Source: CAD feature listing. Evaluate the final solid. Frame: model axes, mm. Face numbers are marked on the shaded views. Coordinates: 2 decimals unless noted, no trailing zeros. Order: outer loops, then holes, each group sorted by start corner. A loop starts at its lowest first (then second) coordinate and runs counter-clockwise, first axis right, second up. Notation, with made-up numbers: (-5, 19.5) -> (32, 19.5) arc R22 cw to (32, 46.5) -> close; hole circle Ø3 at (54.25, -21.5). An arc over 180 degrees is marked (long way). Put each result on its own line as item: value.
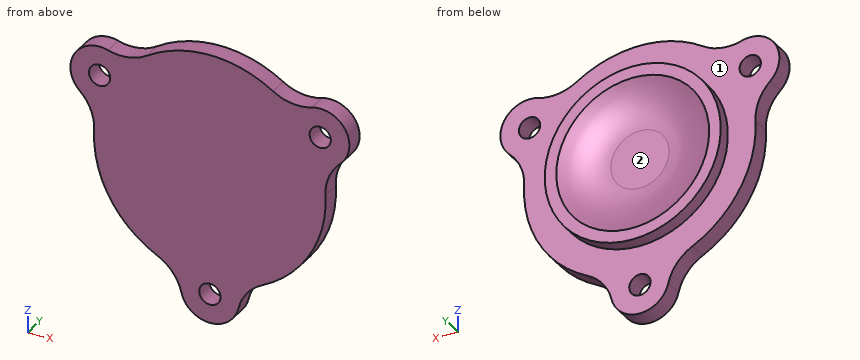
from build123d import *

# Parameters (mm, degrees)
SKETCH_1_R      = 12.5
EXTRUDE_1_DEPTH = 2
SKETCH_2_R      = 9.5
SKETCH_2_R_2    = 8.25
EXTRUDE_2_DEPTH = 1.4
FILLET_1_R      = 10
EXTRUDE_START   = -2
SKETCH_3_R      = 1.15
EXTRUDE_3_DEPTH = 2


with BuildPart() as part:
    # Эскиз1 → Бобышка-Вытянуть1 (new body)
    with BuildSketch(Plane(origin=(0, 0, 0), x_dir=(1, 0, 0), z_dir=(0, 1, 0))):
        with Locations(Location((0, 0, 0), (0, 0, 270))):
            Circle(SKETCH_1_R)
    extrude(amount=EXTRUDE_1_DEPTH)

    # Эскиз2 → Бобышка-Вытянуть2 (add)
    with BuildSketch(Plane(origin=(0, 2, 0), x_dir=(1, 0, 0), z_dir=(0, 1, 0))):
        with Locations(Location((0, 0, 0), (0, 0, 270))):
            Circle(SKETCH_2_R)
        with Locations(Location((0, 0, 0), (0, 0, 270))):
            Circle(SKETCH_2_R_2, mode=Mode.SUBTRACT)
    extrude(amount=EXTRUDE_2_DEPTH)

    # Скругление1
    # the kernel refuses this fillet: 10 mm, written as the material it adds along each edge
    with BuildSketch(Plane(origin=(0, 2, 0), x_dir=(0, 0, 1), z_dir=(-1, 0, 0))) as fillet_1_piece_1:
        with BuildLine():
            CenterArc((3.147059671, 10), FILLET_1_R, 270, 30.683417109)
            Line((3.147059671, 0), (3.147059671, -0.2))
            Line((3.147059671, -0.2), (8.25, -0.2))
            Line((8.25, -0.2), (8.45, 0))
            ThreePointArc((8.45, 0), (8.45, 0.7), (8.352058807, 1.228))
            Line((8.352058807, 1.228), (8.25, 1.4))
        make_face()
    revolve(axis=Axis((0, 2, 0), (0, 1, 0)))

    # Эскиз3 → Бобышка-Вытянуть3 (add)
    # profile 1 of 3: a face of its own
    with BuildSketch(Plane(origin=(0, 2, 0), x_dir=(1, 0, 0), z_dir=(0, 1, 0)).offset(EXTRUDE_START)):
        with BuildLine():
            ThreePointArc((5.670132274, 11.14), (0, 12.5), (-5.670132274, 11.14))
            ThreePointArc((-5.670132274, 11.14), (-4.001241708, 12.51371577), (-3.068132924, 14.463484663))
            ThreePointArc((-3.068132924, 14.463484663), (0, 16.9), (3.068132924, 14.463484663))
            ThreePointArc((3.068132924, 14.463484663), (4.001241708, 12.51371577), (5.670132274, 11.14))
        make_face()
        with Locations(Location((0, 13.75, 0), (0, 0, 270))):
            Circle(SKETCH_3_R, mode=Mode.SUBTRACT)
    # profile 2 of 3: a face of its own
    with BuildSketch(Plane(origin=(0, 2, 0), x_dir=(1, 0, 0), z_dir=(0, 1, 0)).offset(EXTRUDE_START)):
        with BuildLine():
            ThreePointArc((10.991678683, -9.888823385), (14.635829324, -8.45), (14.059811607, -4.574661277))
            ThreePointArc((14.059811607, -4.574661277), (12.837816607, -2.791680919), (12.482589135, -0.659521408))
            ThreePointArc((12.482589135, -0.659521408), (10.825317547, -6.25), (6.812456861, -10.480478592))
            ThreePointArc((6.812456861, -10.480478592), (8.836574899, -9.722034851), (10.991678683, -9.888823385))
        make_face()
        with Locations(Location((11.907849302, -6.875, 0), (0, 0, 270))):
            Circle(SKETCH_3_R, mode=Mode.SUBTRACT)
    # profile 3 of 3: a face of its own
    with BuildSketch(Plane(origin=(0, 2, 0), x_dir=(1, 0, 0), z_dir=(0, 1, 0)).offset(EXTRUDE_START)):
        with BuildLine():
            ThreePointArc((-14.059811607, -4.574661277), (-14.635829324, -8.45), (-10.991678683, -9.888823385))
            ThreePointArc((-10.991678683, -9.888823385), (-8.836574899, -9.722034851), (-6.812456861, -10.480478592))
            ThreePointArc((-6.812456861, -10.480478592), (-10.825317547, -6.25), (-12.482589135, -0.659521408))
            ThreePointArc((-12.482589135, -0.659521408), (-12.837816607, -2.791680919), (-14.059811607, -4.574661277))
        make_face()
        with Locations(Location((-11.907849302, -6.875, 0), (0, 0, 270))):
            Circle(SKETCH_3_R, mode=Mode.SUBTRACT)
    extrude(amount=EXTRUDE_3_DEPTH)


solid = part.part
1. Cut plane B-B on z = -13.75. Output: boundary loops of the cut face in (x, y).
Numbers:
outline: (-3.29, 0) -> (-1.15, 0) -> (-1.15, 2) -> (-3.29, 2) -> close; (1.15, 0) -> (3.29, 0) -> (3.29, 2) -> (1.15, 2) -> close
2. Pull-direction query (Z, two-part tool) for the marked faces 1 and 2; classes: pulls with the +Z half, pulls with the -Z half, needs draft (parallel to the pull), parting line crosses it, or undercut.
Numbers:
face 1: needs draft
face 2: undercut
3. Ray query, line 1 along X through (y, z) = (1.5, 7.5); line 2 along Y through (x, z) = (6.5, -8.5); line 3 along X through (y, z) = (1.3, -13.75). Return the intervals inside material, ascending.
Numbers:
line 1: x = -15 to -12.87, -10.94 to 10.94, 12.87 to 15
line 2: y = 0 to 2
line 3: x = -3.29 to -1.15, 1.15 to 3.29
4. Cut plane A-A on y = 0.7. Output: boundary loops of the cut face in (x, z) (3 decimals).
Numbers:
outline: (-14.06, 4.575) arc R5 cw to (-12.483, 0.66) arc R12.5 ccw to (-5.67, -11.14) arc R5 cw to (-3.068, -14.463) arc R3.15 ccw to (3.068, -14.463) arc R5 cw to (5.67, -11.14) arc R12.5 ccw to (12.483, 0.66) arc R5 cw to (14.06, 4.575) arc R3.15 ccw to (10.992, 9.889) arc R5 cw to (6.812, 10.48) arc R12.5 ccw to (-6.812, 10.48) arc R5 cw to (-10.992, 9.889) arc R3.15 ccw to start; hole circle Ø2.3 at (-11.908, 6.875); hole circle Ø2.3 at (0, -13.75); hole circle Ø2.3 at (11.908, 6.875)
5. First-contact query: pin 1 (3.5 mm diameter, centred on x = -11.91, z = 6.88, fed in from +Y); pin 2 (12 mm diameter, centred on x = -1, z = -11.5, fed in from +Y); pin 3 (1.5 mm diameter, centred on y = 0.5, z = -5, fed in from -X); pin 4 (1 mm diameter, centred on y = 1.5, z = -0.5, fed in from +X). Flat tips, straight axial feed; report the tip coordinate or a pass-through.
Numbers:
pin 1: stops at y = 2
pin 2: stops at y = 3.4
pin 3: stops at x = -11.76
pin 4: stops at x = 12.5
6. Cut plane C-C on z = 7. Count the separate pieces of the cut face and the enclosed holes in it, plus the area to 3 significant figures.
Numbers:
separate pieces: 3
enclosed holes: 0
area: 65.3 mm2
